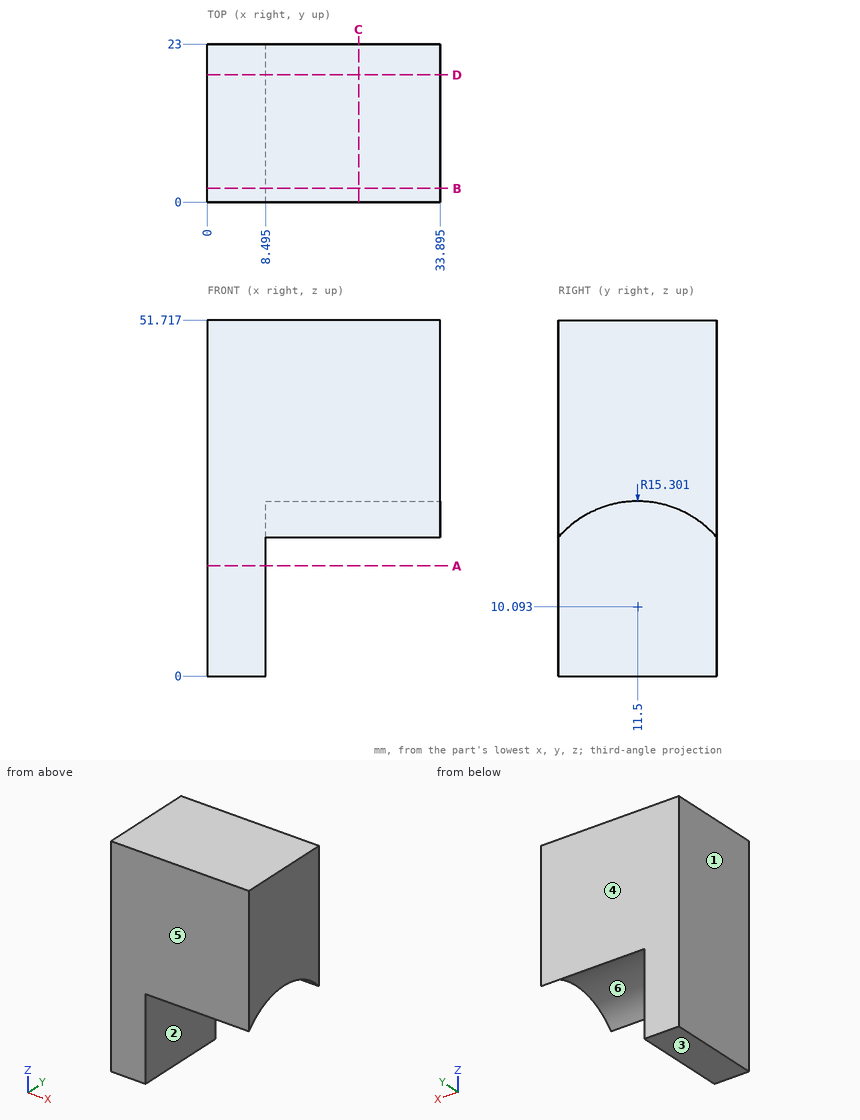
Study the drawing (mm; zero at the part's minimum x, y, z) and answer. A direction names the side the tool comes from. Give positions to 0.01 mm unless a question says otherwise; leave off trailing zeros. Order: outer loops, then holes, each group sorted by start corner. A loop starts at its lowest first (then second) coordinate and runs counter-clockwise, first axis right, second up. Notation, with made-up numbers: (18.5, -29) - (58.5, -29) arc R24 cw to (58.5, 3) - close; hole circle Ø8 at (42.5, 85). An arc over 180 degrees is marked (long way). Answer as CSV lines item,"result". Start each with the question number.
Q1. Find the intervals of material crossed by L1, parallel to X at y = 7.25, z = 10.5 (1 decimal); L2, parallel to Y at x = 9, z = 22; L3, parallel to Z at x = 24, y = 11, in increasing order. Write a range as [from, to].
Q2. For the marked faces 1 and 2, determine the directions among +Z, -Z, +X, -X, +Y, -Y from which every point of the face is accessible in a straight line to the end or side of a thin tool.
Q3. The part is cut by section C-C (x = 22). Write down the section's boundary in (y, z), then the cut area to 3 significant figures.
Q4. The part is cut by section A-A (z = 16). Write down the section's boundary in (x, y) (1 decimal).
Q5. The part is cut by section D-D (y = 18.5). Write down the section's boundary in (x, z) (1 decimal), then the cut area to 3 significant figures.
Q6. The mould has two halves that part along Y. Classify the marked faces 3, 4, 5 and 6: +Y half, -Y half, draft (parallel to the pull), parting line (faces both ways), or undercut.
Q7. Given pin 1 Ø7 at (y, z) = (9, 8) entering from +X (1 decimal); pin 2 Ø5 at (y, z) = (6, 31.5) entering from -X; pin 3 Ø1 at (x, y) = (16, 11) entering from -Z, each flat-ended and moving along its own axis, determine where each tip first touches the part or whether it passes through.
Q8. The part is cut by section B-B (y = 2). Write down the section's boundary in (x, z) (1 decimal).
Check result:
1,L1,"x = [0, 8.5]"
1,L2,"y = [0, 1.89], [21.11, 23]"
1,L3,"z = [25.39, 51.72]"
2,face 1,"+Z, -Z, -X, +Y, -Y"
2,face 2,"-Z, +X"
3,outline,"(0, 20.19) arc R15.3 cw to (23, 20.19) - (23, 51.72) - (0, 51.72) - close"
3,area,"642 mm²"
4,outline,"(0, 0) - (8.5, 0) - (8.5, 23) - (0, 23) - close"
5,outline,"(0, 0) - (8.5, 0) - (8.5, 23.7) - (33.9, 23.7) - (33.9, 51.7) - (0, 51.7) - close"
5,area,"1,150 mm²"
6,face 3,"draft"
6,face 4,"+Y half"
6,face 5,"-Y half"
6,face 6,"undercut"
7,pin 1,"stops at x = 8.5"
7,pin 2,"stops at x = 0"
7,pin 3,"stops at z = 25.36"
8,outline,"(0, 0) - (8.5, 0) - (8.5, 22.1) - (33.9, 22.1) - (33.9, 51.7) - (0, 51.7) - close"
